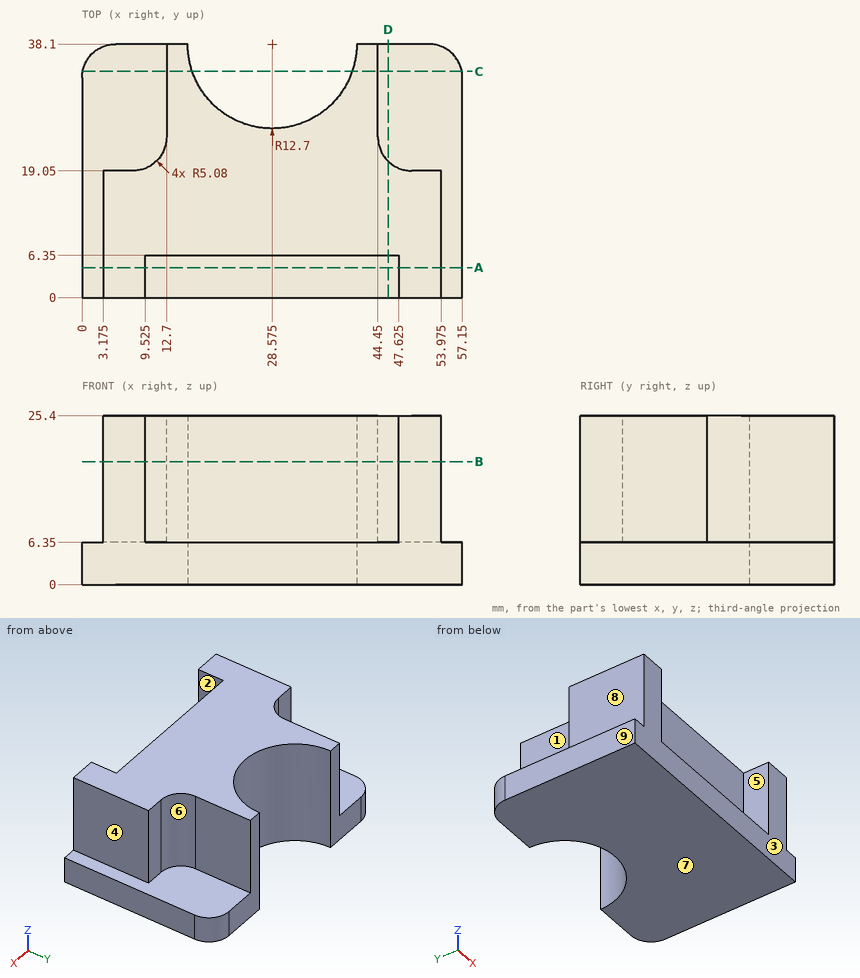
Print and shaded views of the part. All mm, measured from the part's lowest x, y and z. A direction names the side the tool comes from. Coordinates: 2 decimals unless noted, no trailing zeros. Order: outer loops, then holes, each group sorted by start corner. A loop starts at its lowest first (then second) coordinate and runs counter-clockwise, first axis right, second up.
(1) Pin check, flat tips, straight feed: pin 1 Ø1.5 at (x, z) = (17, 14) entering from -Y; pin 2 Ø2 at (x, z) = (52, 18.5) entering from +Y; pin 3 Ø9.5 at (y, z) = (7, 19.5) entering from -X (3 decimals). Stop position of each tip, or through.
Check sheet entries:
pin 1: stops at y = 6.35
pin 2: stops at y = 19.05
pin 3: stops at x = 3.175
(2) Slice it at D-D, the plane x = 46. Write the cut outline in (y, z), and give its area (3 significant figures).
Check sheet entries:
outline: (0, 0) - (38.1, 0) - (38.1, 6.35) - (20.48, 6.35) - (20.48, 25.4) - (6.35, 25.4) - (6.35, 6.35) - (0, 6.35) - close
area: 511 mm2
(3) Slice it at B-B, the plane z = 18.5. Write the cut outline in (x, y) (3 decimals).
Check sheet entries:
outline: (3.175, 0) - (9.525, 0) - (9.525, 6.35) - (47.625, 6.35) - (47.625, 0) - (53.975, 0) - (53.975, 19.05) - (49.53, 19.05) arc R5.08 cw to (44.45, 24.13) - (44.45, 38.1) - (41.275, 38.1) arc R12.7 cw to (15.875, 38.1) - (12.7, 38.1) - (12.7, 24.13) arc R5.08 cw to (7.62, 19.05) - (3.175, 19.05) - close
(4) Probe L1, parallel to X at y = 2, z = 22.25 (3 decimals); L2, parallel to X at y = 17, z = 17.25 (3 decimals); L3, parallel to Y at x = 5, z = 7. List the from-to ranges inside material, lowest first.
Check sheet entries:
L1: x = 3.175 to 9.525, 47.625 to 53.975
L2: x = 3.175 to 53.975
L3: y = 0 to 19.05
(5) Slice it at C-C, the plane y = 34. Write the cut outline in (x, z).
Check sheet entries:
outline: (0.1, 0) - (16.56, 0) - (16.56, 25.4) - (12.7, 25.4) - (12.7, 6.35) - (0.1, 6.35) - close; (40.59, 0) - (57.05, 0) - (57.05, 6.35) - (44.45, 6.35) - (44.45, 25.4) - (40.59, 25.4) - close
(6) Slice it at A-A, the plane y = 4.5. Write the cut outline in (x, z) (3 decimals).
Check sheet entries:
outline: (0, 0) - (57.15, 0) - (57.15, 6.35) - (53.975, 6.35) - (53.975, 25.4) - (47.625, 25.4) - (47.625, 6.35) - (9.525, 6.35) - (9.525, 25.4) - (3.175, 25.4) - (3.175, 6.35) - (0, 6.35) - close
(7) Tool access for the marked faces 5, 6, 7, 8 and 9: list every direction of +Z, -Z, +X, -X, +Y, -Y with a clear straight run to the whole face (end or side of a thin tool).
Check sheet entries:
face 5: +Z, -Y
face 6: +Z, +X, +Y
face 7: -Z, +X, -X, +Y, -Y
face 8: +Z, -X, +Y, -Y
face 9: +Z, -Z, -X, +Y, -Y
(8) Pull direction X, two halves, no side cores. Call the marked faces 1, 2, 3 and 4: pulls with the +X half, pulls with the -X half, needs draft (parallel to the pull), parting line crosses it, or undercut.
Check sheet entries:
face 1: pulls with the -X half
face 2: undercut
face 3: needs draft
face 4: pulls with the +X half
